Drawing for the job (mm, zero at the part's lowest x, y, z). A direction names the side the tool comes from. Give positions to 0.01 mm unless a question says otherwise; leave off trailing zeros. Write each loop counter-clockwise with the first axis right and the second up, starting at its lowest first coordinate (ties: lowest second). Pieces come first, ordered by that corner, then holes. Notation, with made-up numbers: (51.5, 61.5) - (77.5, 61.5) arc R26 cw to (77.5, 100.5) - close; hole circle Ø3 at (72, -21). An arc over 180 degrees is marked (long way). Write item = value, one per line. Start each with the question number.
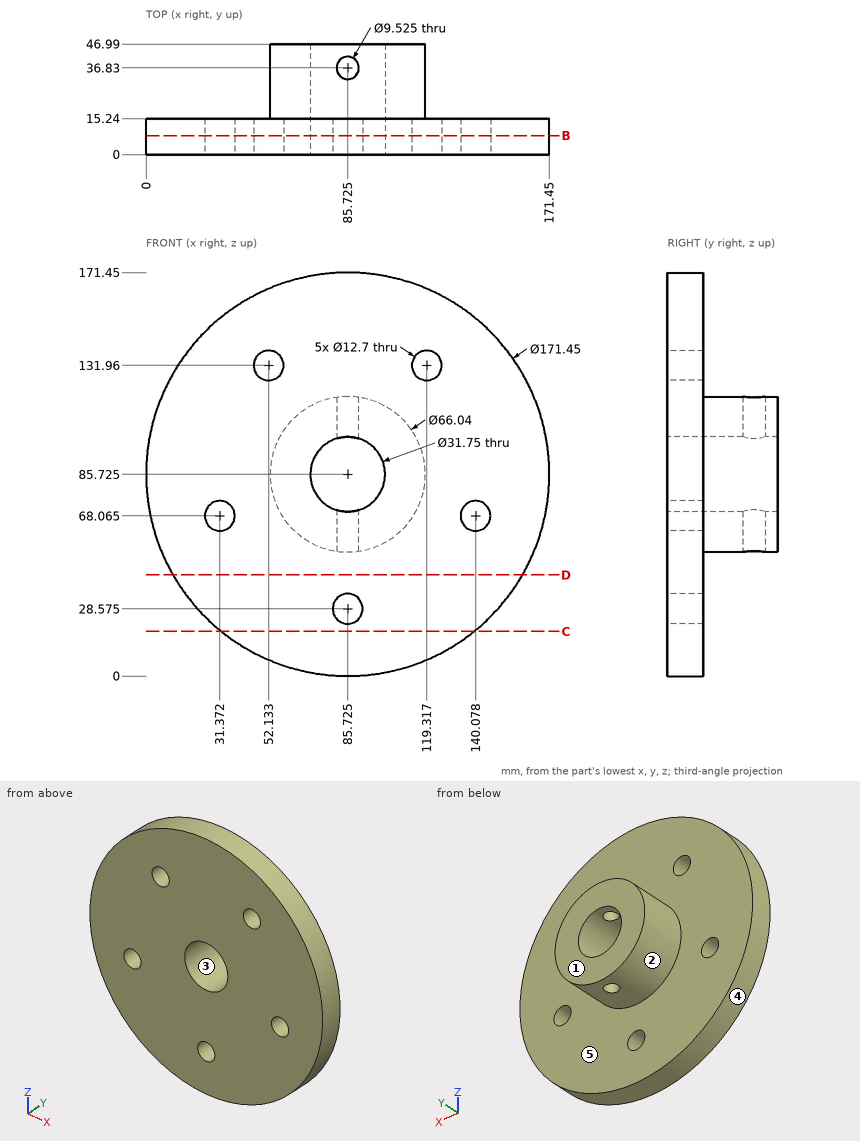
1. Wall check: line 1 along X through (y, z) = (9, 72.5) (1 decimal); line 2 along Y through (x, z) = (68.5, 153); line 3 along Z through (x, y) = (33.5, 7) (1 decimal). Give the ranges that are in metal, low to high.
2. Cut at C-C (z = 19). Give the cut face in (x, y) (1 decimal).
3. Cut at D-D (z = 43). Give the cut face in (x, y), then the cut area to 3 significant figures.
4. Tool access for the marked faces 4 and 5: list every direction of +Z, -Z, +X, -X, +Y, -Y with a clear straight run to the whole face (end or side of a thin tool).
5. Pin check, flat tips, straight feed: pin 1 Ø14.5 at (x, z) = (140.08, 68.06) entering from +Y; pin 2 Ø5 at (x, y) = (102.5, 25) entering from -Z; pin 3 Ø5 at (y, z) = (8.5, 51.5) entering from +X. Stop position of each tip, or through.
6. Mould opens along Z. For the marked faces 1, 2 and 3 say: +Z half, -Z half, draft (parallel to the pull), parting line (faces both ways), or undercut.
7. Cut at B-B (y = 8). Count the separate pieces of the cut face and the enclosed holes in it, then the cut area to 3 significant figures.
Output:
q1.line_1 = 1 to 26.8, 35.9 to 76.9, 94.5 to 135.5, 144.6 to 170.4
q1.line_2 = 0 to 15.24
q1.line_3 = 17.7 to 62.1, 74 to 153.7
q2.outline = (31.9, 0) - (139.5, 0) - (139.5, 15.2) - (31.9, 15.2) - close
q3.outline = (11.41, 0) - (160.04, 0) - (160.04, 15.24) - (11.41, 15.24) - close
q3.area = 2,270 mm2
q4.face_4 = +Y, -Y
q4.face_5 = +Y
q5.pin_1 = 15.24
q5.pin_2 = 55.95
q5.pin_3 = 165.36
q6.face_1 = draft
q6.face_2 = parting line
q6.face_3 = undercut
q7.separate_pieces = 1
q7.enclosed_holes = 6
q7.area = 21,700 mm2
